Could you check a few things on this model? Use its own coordinates, in mm. A direction names the side the tool comes from. Give positions to 0.01 mm unless a question says otherwise; leave off trailing zeros. Loops run counter-clockwise (first coordinate to the right, second up) from the corner with the lowest first, then second, coordinate; pieces in that order, holes last. Notation, with made-up numbers: M -13.5,-6.75 L 10.5,-6.75 A22 ccw 10.5,2.25 Z; hole C 67,-30 d8. An arc over 180 degrees is marked long. Answer in a Markdown table with one row per item. Add a question column.
```python
from build123d import *

# Parameters (mm, degrees)
F0_W     = 127
F0_H     = 127
F1_DEPTH = 63.5
F2_R     = 50.8
F3_DEPTH = 12.7
F4_R     = 38.1
F5_DEPTH = 12.7
F6_R     = 25.4
F7_DEPTH = 12.7
F8_R     = 12.7
F9_DEPTH = 12.7


with BuildPart() as f1:
    # F0 (on Front) → F1 (new body, symmetric)
    with BuildSketch(Plane.XZ):
        Rectangle(F0_W, F0_H)
    extrude(amount=F1_DEPTH, both=True)

    # F2 (on face) → F3 (cut)
    with BuildSketch(Plane.XY.offset(63.5)):
        Circle(F2_R)
    extrude(amount=-F3_DEPTH, mode=Mode.SUBTRACT)

    # F4 (on face) → F5 (cut)
    with BuildSketch(Plane.XY.offset(50.8)):
        Circle(F4_R)
    extrude(amount=-F5_DEPTH, mode=Mode.SUBTRACT)

    # F6 (on face) → F7 (cut)
    with BuildSketch(Plane.XY.offset(38.1)):
        Circle(F6_R)
    extrude(amount=-F7_DEPTH, mode=Mode.SUBTRACT)

    # F8 (on face) → F9 (cut)
    with BuildSketch(Plane.XY.offset(25.4)):
        Circle(F8_R)
    extrude(amount=-F9_DEPTH, mode=Mode.SUBTRACT)


solid = f1.part
```
Item 1: Suppose I cut it at C-C (x = 15.5). List the corners of the cut face in (y, z) for me.
Item 2: For faces 1 (the face through (-1, -63.5, 1)), 2 (the face through (7, 38, 50.8)), which set-ups out of +Z, -Z, +X, -X, +Y, -Y let a thin tool reach every point of the face, with its end or its side?
Item 3: Suppose I cut it at D-D (y = -29). List the corners of the cut face in (x, z) for me.
Item 4: For P1, Ø4, axis at x = 6, y = -24, coming from the +Z side; P2, Ø12.5, axis at x = -5, y = 4.5, coming from the +Z side, each with a flat end and sliding along its axis, tell me the tip position at first contact or that it passes through.
Item 5: If we mould it in two halves opening along X, with no side actions, what happens to faces 3 (the face through (-30.235, -23.183, 44.539)), 4 (the face through (63.5, -1, -1)), 5 (the face through (5, 12, 25.4)), 6 (the face through (-1, -1, -63.5))? For each: +X half, -X half, draft (parallel to the pull), parting line (faces both ways), or undercut.
Item 6: I need wall thicknesses on L1, parallel to X at y = -1, z = 56; L2, parallel to Y at x = 0, z = 17; L3, parallel to Z at x = 0.5, y = 6.5. Which ranges of each line are inside material? Lowest first, please.
Item 7: Suppose I cut it at A-A (y = 0). List the corners of the cut face in (x, z) for me.
Values found:
| question | item | result |
|---|---|---|
| 1 | outline | M -63.5,-63.5 L 63.5,-63.5 L 63.5,63.5 L 48.38,63.5 L 48.38,50.8 L 34.8,50.8 L 34.8,38.1 L 20.12,38.1 L 20.12,25.4 L -20.12,25.4 L -20.12,38.1 L -34.8,38.1 L -34.8,50.8 L -48.38,50.8 L -48.38,63.5 L -63.5,63.5 Z |
| 2 | face 1 | +Z, -Z, +X, -X, -Y |
| 2 | face 2 | +Z |
| 3 | outline | M -63.5,-63.5 L 63.5,-63.5 L 63.5,63.5 L 41.71,63.5 L 41.71,50.8 L 24.71,50.8 L 24.71,38.1 L -24.71,38.1 L -24.71,50.8 L -41.71,50.8 L -41.71,63.5 L -63.5,63.5 Z |
| 4 | P1 | z = 38.1 |
| 4 | P2 | z = 25.4 |
| 5 | face 3 | undercut |
| 5 | face 4 | +X half |
| 5 | face 5 | undercut |
| 5 | face 6 | draft |
| 6 | L1 | -63.5 to -50.79, 50.79 to 63.5 |
| 6 | L2 | -63.5 to -12.7, 12.7 to 63.5 |
| 6 | L3 | -63.5 to 12.7 |
| 7 | outline | M -63.5,-63.5 L 63.5,-63.5 L 63.5,63.5 L 50.8,63.5 L 50.8,50.8 L 38.1,50.8 L 38.1,38.1 L 25.4,38.1 L 25.4,25.4 L 12.7,25.4 L 12.7,12.7 L -12.7,12.7 L -12.7,25.4 L -25.4,25.4 L -25.4,38.1 L -38.1,38.1 L -38.1,50.8 L -50.8,50.8 L -50.8,63.5 L -63.5,63.5 Z |
